For this review, take the finished solid that the model builds, in its own axes (mm). A direction names the side the tool comes from. Round coordinates to 2 decimals unless told otherwise and drop trailing zeros. Order: outer loops, then holes, each group sorted by start corner. A loop starts at its lowest first (then second) coordinate and runs counter-clockwise, first axis right, second up. Notation, with made-up numbers: (36, -26) - (68, -26) arc R21 ccw to (68, 6) - close; hole circle Ø4 at (25.5, 29.25). An arc over 180 degrees is marked (long way). One line per question, with ' | ' between items.
```python
from build123d import *

# Parameters (mm, degrees)
F0_R     = 73.025
F0_R_2   = 7.62
F1_DEPTH = 12.7
F2_R     = 5.08
F3_DEPTH = 19.05


with BuildPart() as f1:
    # F0 (on Front) → F1 (new body)
    with BuildSketch(Plane.XZ):
        Circle(F0_R)
        with Locations((-34.87542, 39.516099)):
            Circle(F0_R_2, mode=Mode.SUBTRACT)
    extrude(amount=F1_DEPTH)

    # F2
    f2_edges = [f1.edges().sort_by_distance(p)[0] for p in [
        (-73.025, -12.7, 0),
    ]]
    fillet(f2_edges, radius=F2_R)

    # F0 (on Front) → F3 (join)
    with BuildSketch(Plane.XZ):
        with Locations((-34.87542, 39.516099)):
            Circle(F0_R_2)
    extrude(amount=F3_DEPTH)


solid = f1.part
```
(1) We need section D-D on y = -16.5. State the section outline as (x, z) points, plus the area to 3 significant figures.
Output values:
outline: circle Ø15.24 at (-34.88, 39.52) | area: 182 mm^2
(2) For faces 1 (the flat face through (-35, -19.05, 40)), 2 (the cylindrical face through (-40.49, -15.83, 44.67)), list the 3-axis set-ups (+Z, -Z, +X, -X, +Y, -Y) from which the entire face can be reached by the end or side of a thin tool; tool diameter is ignored.
Output values:
face 1: +Z, -Z, +X, -X, -Y | face 2: -Y
(3) We need section A-A on y = -2. State the section outline as (x, z) points (3 decimals), plus the area to 3 significant figures.
Output values:
outline: circle Ø146.05 at (0, 0) | area: 16,800 mm^2
(4) We need section C-C on x = 0. State the section outline as (y, z) points (3 decimals).
Output values:
outline: (-12.7, -67.945) arc R5.08 ccw to (-7.62, -73.025) - (0, -73.025) - (0, 73.025) - (-7.62, 73.025) arc R5.08 ccw to (-12.7, 67.945) - close
(5) Insertion check: pin 1 (3 mm diameter, centred on x = 33.5, y = -8, fed in from +Z); pin 2 (1.5 mm diameter, centred on x = 40.5, y = -6, fed in from +Z); pin 3 (1.5 mm diameter, centred on x = 49, y = -6, fed in from +Z); pin 4 (4 mm diameter, centred on x = 3.5, z = -20, fed in from +Y). Each pin has a flat end and moves straight along its axis. Give the tip position at first contact, or say it passes through.
Output values:
pin 1: z = 65.63 | pin 2: z = 61.26 | pin 3: z = 54.81 | pin 4: y = 0
(6) We need section B-B on z = 0. State the section outline as (x, y) points (3 decimals), plus the area to 3 significant figures.
Output values:
outline: (-73.025, -7.62) arc R5.08 ccw to (-67.945, -12.7) - (67.945, -12.7) arc R5.08 ccw to (73.025, -7.62) - (73.025, 0) - (-73.025, 0) - close | area: 1,840 mm^2
(7) For probe 1 along Y at (x, z) = (12, -23); probe 2 along Z at (x, y) = (23, -7.5); probe 3 along Z at (x, y) = (-30.5, -3.5), list the stretches that pass through material, from the lowest coordinate up. Write a range as [from, to].
Output values:
probe 1: [-12.7, 0] | probe 2: [-69.31, 69.31] | probe 3: [-66.35, 66.35]
